from build123d import *

# Parameters (mm, degrees)
F0_W      = 20
F0_H      = 20
F1_DEPTH  = 5
F2_W      = 12
F2_H      = 12
F2_W_2    = 9
F2_H_2    = 9
F3_DEPTH  = 5
F5_D      = 16.5
F5_DEPTH  = 3
F5_TIP    = 4.957100107
F6_W      = 20
F6_H      = 4
F7_DEPTH  = 5
F9_DEPTH  = 20.001
F11_DEPTH = 20


with BuildPart() as f1:
    # F0 (on Front) → F1 (new body)
    with BuildSketch(Plane.XZ):
        Rectangle(F0_W, F0_H)
    extrude(amount=F1_DEPTH)

    # F2 (on face) → F3 (join)
    with BuildSketch(Plane.XZ.offset(5)):
        Rectangle(F2_W, F2_H)
        Rectangle(F2_W_2, F2_H_2, mode=Mode.SUBTRACT)
    extrude(amount=F3_DEPTH)

    # F5
    with Locations(Plane(origin=(0, 0, 0), x_dir=(-1, 0, 0), z_dir=(0, 1, 0))):
        with Locations((0, 0)):
            Hole(F5_D / 2, depth=F5_DEPTH)
            with Locations((0, 0, -(F5_DEPTH + F5_TIP / 2))):  # 118° drill point
                Cone(0, F5_D / 2, F5_TIP, mode=Mode.SUBTRACT)

    # F6 (on face) → F7 (join)
    with BuildSketch(Plane.XZ.offset(5)):
        with Locations((0, -8)):
            Rectangle(F6_W, F6_H)
    extrude(amount=F7_DEPTH)

    # F8 (on face) → F9 (cut, through all)
    with BuildSketch(Plane(origin=(-10, 0, 0), x_dir=(0, -1, 0), z_dir=(-1, 0, 0))):
        Polygon((10, -6), (5, -10), (10, -10), align=None)
    extrude(amount=-F9_DEPTH, mode=Mode.SUBTRACT)

    # F10 (on face) → F11 (join)
    with BuildSketch(Plane(origin=(-10, 0, 0), x_dir=(0, -1, 0), z_dir=(-1, 0, 0))):
        Polygon((0, -14), (5, -10), (0, -10), align=None)
    extrude(amount=-F11_DEPTH)


solid = f1.part
Design review of the part built by this model. Coordinates are the model's own, in mm. A direction names the side the tool comes from. Give positions to 0.01 mm unless a question says otherwise; leave off trailing zeros. Order: outer loops, then holes, each group sorted by start corner. A loop starts at its lowest first (then second) coordinate and runs counter-clockwise, first axis right, second up. Notation, with made-up numbers: (19, 25.25) - (73, 25.25) arc R19 cw to (73, 51.25) - close; hole circle Ø3 at (9, 3). An arc over 180 degrees is marked (long way). Use CSV: the item, a comma, the result in double quotes. Start each with the question number.
Q1. Take a section at D-D (y = -6.5). State the section outline as (x, z) points, and give its area (3 significant figures).
Q2. Take a section at C-C (y = -8.5). State the section outline as (x, z) points, and give its area (3 significant figures).
Q3. Take a section at A-A (z = 0). State the section outline as (x, y) points, and give its area (3 significant figures).
Q4. For line 1 (X direction, y = -2.1, z = 0); line 2 (X direction, y = -7.25, z = -2); line 3 (Z direction, x = -2, y = -2), list the stretches that pass through material, from the lowest coordinate up.
Q5. For P1, Ø1.2, axis at x = -9, y = -7.5, coming from the +Z side; P2, Ø3, axis at x = 5.5, z = -6.5, coming from the +Y side; P3, Ø6, axis at x = 2.5, z = -0.5, coming from the +Y side; P4, Ø1.5, axis at x = -0.5, y = -6.5, coming from the +Z side, all flat-tipped, find the tip position at first contact; note any pin that passes through.
Q6. Draft analysis for pull direction Z (two halves, no side actions). For faces 5 (the face through (0, -7, 6)), 6 (the face through (-6, -7, 0)), 7 (the face through (7.62, -1.52, -3.16)), state which applies: pulls with the +Z half, pulls with the -Z half, needs draft (parallel to the pull), parting line crosses it, or undercut.
Q7. Take a section at B-B (x = 0). State the section outline as (y, z) points.
Q8. Machinability: for faces 1 (the face through (10, -3, -2)), 2 (the face through (8, -7, -6)), 3 (the face through (0, -7, -4.5)), 4 (the face through (-8, -7, -6)), which of the approach directions +Z, -Z, +X, -X, +Y, -Y give a long, thin tool a straight path to every point of the face, cutting with its end or side? Answer none if there is none.
Calculated:
1,outline,"(-10, -8.8) - (10, -8.8) - (10, -6) - (6, -6) - (6, 6) - (-6, 6) - (-6, -6) - (-10, -6) - close; hole (-4.5, -4.5) - (4.5, -4.5) - (4.5, 4.5) - (-4.5, 4.5) - close"
1,area,"119 mm²"
2,outline,"(-10, -7.2) - (10, -7.2) - (10, -6) - (6, -6) - (6, 6) - (-6, 6) - (-6, -6) - (-10, -6) - close; hole (-4.5, -4.5) - (4.5, -4.5) - (4.5, 4.5) - (-4.5, 4.5) - close"
2,area,"87.0 mm²"
3,outline,"(-10, -5) - (-6, -5) - (-6, -10) - (-4.5, -10) - (-4.5, -5.25) - (-8.25, -3) - (-8.25, 0) - (-10, 0) - close; (4.5, -10) - (6, -10) - (6, -5) - (10, -5) - (10, 0) - (8.25, 0) - (8.25, -3) - (4.5, -5.25) - close"
3,area,"39.1 mm²"
4,line 1,"x = -10 to -8.25, 8.25 to 10"
4,line 2,"x = -6 to -4.5, 4.5 to 6"
4,line 3,"z = -12.4 to -8, 8 to 10"
5,P1,"stops at z = -6"
5,P2,"stops at y = 0"
5,P3,"stops at y = -4.62"
5,P4,"stops at z = 6"
6,face 5,"pulls with the +Z half"
6,face 6,"needs draft"
6,face 7,"undercut"
7,outline,"(-10, -6) - (0, -14) - (0, -8.25) - (-3, -8.25) - (-5.25, -4.5) - (-10, -4.5) - close; (-10, 4.5) - (-5.25, 4.5) - (-3, 8.25) - (0, 8.25) - (0, 10) - (-5, 10) - (-5, 6) - (-10, 6) - close"
8,face 1,"+Z, -Z, +X, +Y, -Y"
8,face 2,"+Z, +X, -Y"
8,face 3,"-Y"
8,face 4,"+Z, -X, -Y"
